from build123d import *

# Parameters (mm, degrees)
SKETCH_1_R          = 50
SKETCH_1_R_2        = 48
EXTRUDE_1_DEPTH     = 385
CUT_EXTRUDE_START   = -8
CUT_EXTRUDE_1_DEPTH = 8
FILLET_1_R          = 0.5
FILLET_2_R          = 1


with BuildPart() as part:
    # Эскиз1 → Бобышка-Вытянуть1 (new body)
    with BuildSketch(Plane.XY):
        Circle(SKETCH_1_R)
        Circle(SKETCH_1_R_2, mode=Mode.SUBTRACT)
    extrude(amount=EXTRUDE_1_DEPTH)

    # Эскиз3 → Вырез-Вытянуть1 (cut)
    with BuildSketch(Plane.XY.offset(385).offset(CUT_EXTRUDE_START)):
        with BuildLine():
            Line((-1.92, -47.961584628), (-2, -49.959983987))
            ThreePointArc((-2, -49.959983987), (0, -50), (2, -49.959983987))
            Line((2, -49.959983987), (1.92, -47.961584628))
            ThreePointArc((1.92, -47.961584628), (0, -48), (-1.92, -47.961584628))
        make_face()
    cut_extrude_1 = extrude(amount=CUT_EXTRUDE_1_DEPTH, mode=Mode.SUBTRACT)

    # Зеркальное отражение3: Вырез-Вытянуть1 across plane
    add(cut_extrude_1.mirror(Plane.XY.offset(192.5)), mode=Mode.SUBTRACT)

    # Скругление1
    fillet_1_edges = [part.edges().sort_by_distance(p)[0] for p in [
        (-1.96, -48.960784307, 377),
        (1.96, -48.960784307, 377),
        (1.96, -48.960784307, 8),
        (-1.96, -48.960784307, 8),
    ]]
    fillet(fillet_1_edges, radius=FILLET_1_R)

    # Скругление2
    fillet_2_edges = [part.edges().sort_by_distance(p)[0] for p in [
        (1.96, -48.960784307, 385),
        (-1.96, -48.960784307, 385),
        (1.96, -48.960784307, 0),
        (-1.96, -48.960784307, 0),
    ]]
    fillet(fillet_2_edges, radius=FILLET_2_R)


solid = part.part
Could you check a few things on this model? Use its own coordinates, in mm. Coordinates: 2 decimals unless noted, no trailing zeros. Write each loop counter-clockwise with the first axis right and the second up, starting at its lowest first coordinate (ties: lowest second). Pieces come first, ordered by that corner, then holes. Notation, with made-up numbers: M 7.5,52.25 L 17.5,52.25 A14 ccw 17.5,78.25 Z; hole C 31.25,32.25 d4. An arc over 180 degrees is marked long. One line per question, with ' | ' between items.
1) Imagine slicing it at A-A, the plane y = 0. Write out the boundary of the cut face in (x, z), and give its area (3 significant figures).
Checks:
outline: M -50,0 L -48,0 L -48,385 L -50,385 Z; M 48,0 L 50,0 L 50,385 L 48,385 Z | area: 1,540 mm²
2) Imagine slicing it at C-C, the plane z = 307. Write out the boundary of the cut face in (x, y).
Checks:
outline: C 0,0 d100; hole C 0,0 d96
3) For pin 1 Ø6 at (x, z) = (26, 175.5) entering from +Y; pin 2 Ø3 at (x, z) = (-8.5, 148.5) entering from -Y; pin 3 Ø3 at (y, z) = (5, 191.5) entering from -X, each with a flat end and sliding along its axis, tell me the tip position at first contact or that it passes through.
Checks:
pin 1: y = 44.4 | pin 2: y = -49.51 | pin 3: x = -49.88
4) I need wall thicknesses on probe 1 along Y at (x, z) = (0, 158); probe 2 along Y at (x, z) = (-15, 290). Which ranges of each line are inside material? Lowest first, please. Write a range as [from, to].
Checks:
probe 1: [-50, -48], [48, 50] | probe 2: [-47.7, -45.6], [45.6, 47.7]
5) Imagine slicing it at B-B, the plane x = 16. Write out the boundary of the cut face in (y, z).
Checks:
outline: M -47.37,0 L -45.25,0 L -45.25,385 L -47.37,385 Z; M 45.25,0 L 47.37,0 L 47.37,385 L 45.25,385 Z
